from build123d import *

# Parameters (mm, degrees)
SKETCH_3_R          = 23.4
EXTRUDE_1_DEPTH     = 7.81
SKETCH_2_R          = 21.6
CUT_EXTRUDE_1_DEPTH = 2.1
CUT_EXTRUDE_START   = 2.1
CUT_EXTRUDE_2_DEPTH = 3.2
CUT_EXTRUDE_START_2 = 7.81
SKETCH_4_R          = 1.49999954
SKETCH_4_R_2        = 1.25000004
CUT_EXTRUDE_5_DEPTH = 8.81
SKETCH_5_R          = 1.65
CUT_EXTRUDE_6_DEPTH = 0.9
SKETCH_6_R          = 2.35
CUT_EXTRUDE_7_DEPTH = 2.7
CUT_EXTRUDE_START_3 = 5.3
SKETCH_7_R          = 3.2
CUT_EXTRUDE_8_DEPTH = 1
CHAMFER_1_SIZE      = 1
CHAMFER_2_SIZE      = 0.25
CHAMFER_3_SIZE      = 0.2


with BuildPart() as part:
    # 草图3 → 凸台-拉伸1 (new body)
    with BuildSketch(Plane.XY):
        with Locations((100.000148425, 100.000129687)):
            Circle(SKETCH_3_R)
    extrude(amount=EXTRUDE_1_DEPTH)

    # 草图2 → 切除-拉伸1 (cut)
    with BuildSketch(Plane.XY):
        with Locations((100.000148425, 100.000129687)):
            Circle(SKETCH_2_R)
    extrude(amount=CUT_EXTRUDE_1_DEPTH, mode=Mode.SUBTRACT)

    # 草图1 → 切除-拉伸2 (cut)
    with BuildSketch(Plane.XY.offset(CUT_EXTRUDE_START)):
        with BuildLine():
            Line((112.259115553, 115.826027875), (111.656637713, 115.826027875))
            Line((111.656637713, 115.826027875), (97.599477613, 115.826027875))
            Line((97.599477613, 115.826027875), (96.687659742, 115.826027875))
            ThreePointArc((96.687659742, 115.826027875), (96.087351408, 115.611111205), (95.759847053, 115.064027875))
            Line((95.759847053, 115.064027875), (95.759847053, 109.857027875))
            Line((95.759847053, 109.857027875), (95.759847053, 105.158027875))
            ThreePointArc((95.759847053, 105.158027875), (95.387872666, 104.260002263), (94.489847053, 103.888027875))
            Line((94.489847053, 103.888027875), (83.186847053, 103.888027875))
            ThreePointArc((83.186847053, 103.888027875), (82.288821441, 103.516053487), (81.916847053, 102.618027875))
            Line((81.916847053, 102.618027875), (81.916847053, 92.712027875))
            ThreePointArc((81.916847053, 92.712027875), (82.288821441, 91.814002263), (83.186847053, 91.442027875))
            Line((83.186847053, 91.442027875), (92.965847053, 91.442027875))
            ThreePointArc((92.965847053, 91.442027875), (94.021841281, 91.231977601), (94.917069973, 90.633804955))
            Line((94.917069973, 90.633804955), (95.676425833, 89.874449095))
            ThreePointArc((95.676425833, 89.874449095), (96.208135359, 89.078689918), (96.394847053, 88.140027875))
            Line((96.394847053, 88.140027875), (96.394847053, 81.461633815))
            ThreePointArc((96.394847053, 81.461633815), (96.427853197, 81.29569991), (96.521847053, 81.155027875))
            ThreePointArc((96.521847053, 81.155027875), (96.943861908, 80.87304655), (97.441662377, 80.774027875))
            Line((97.441662377, 80.774027875), (97.537847053, 80.774027875))
            Line((97.537847053, 80.774027875), (101.772425833, 80.774027875))
            Line((101.772425833, 80.774027875), (102.236847053, 80.774027875))
            ThreePointArc((102.236847053, 80.774027875), (102.865464982, 81.034409947), (103.125847053, 81.663027875))
            Line((103.125847053, 81.663027875), (103.125847053, 83.695027875))
            ThreePointArc((103.125847053, 83.695027875), (103.349031686, 84.233843243), (103.887847053, 84.457027875))
            Line((103.887847053, 84.457027875), (111.60403053, 84.457027875))
            ThreePointArc((111.60403053, 84.457027875), (112.336497489, 84.602724612), (112.957452993, 85.017633815))
            Line((112.957452993, 85.017633815), (117.811624454, 89.871805276))
            ThreePointArc((117.811624454, 89.871805276), (118.408450098, 90.766392606), (118.618000745, 91.821179725))
            Line((118.618000745, 91.821179725), (118.618000745, 108.839))
            Line((118.618000745, 108.839), (118.618000745, 109.460547459))
            ThreePointArc((118.618000745, 109.460547459), (118.537945969, 109.810671539), (118.33936792, 110.109941312))
            Line((118.33936792, 110.109941312), (117.729, 110.744000093))
            Line((117.729, 110.744000093), (115.585546543, 112.887726165))
            ThreePointArc((115.585546543, 112.887726165), (114.325244429, 114.275507158), (112.941853583, 115.540626625))
            ThreePointArc((112.941853583, 115.540626625), (112.628834267, 115.751145515), (112.259115553, 115.826027875))
        make_face()
    extrude(amount=CUT_EXTRUDE_2_DEPTH, mode=Mode.SUBTRACT)

    # 草图4 → 切除-拉伸5 (cut, through all)
    with BuildSketch(Plane.XY.offset(CUT_EXTRUDE_START_2)):
        with Locations((85.217, 99.949)):
            Circle(SKETCH_4_R)
        with Locations((93.13750232, 88.11380142)):
            Circle(SKETCH_4_R_2)
        with Locations((93.13749978, 111.8861999)):
            Circle(SKETCH_4_R_2)
    extrude(amount=-CUT_EXTRUDE_5_DEPTH, mode=Mode.SUBTRACT)

    # 草图5 → 切除-拉伸6 (cut)
    with BuildSketch(Plane.XY.offset(CUT_EXTRUDE_START_2)):
        with Locations((85.217, 99.949)):
            Circle(SKETCH_5_R)
    extrude(amount=-CUT_EXTRUDE_6_DEPTH, mode=Mode.SUBTRACT)

    # 草图6 → 切除-拉伸7 (cut)
    with BuildSketch(Plane.XY.offset(CUT_EXTRUDE_START_2)):
        with Locations((93.13749978, 111.8861999)):
            Circle(SKETCH_6_R)
        with Locations((93.13750232, 88.11380142)):
            Circle(SKETCH_6_R)
    extrude(amount=-CUT_EXTRUDE_7_DEPTH, mode=Mode.SUBTRACT)

    # 草图7 → 切除-拉伸8 (cut)
    with BuildSketch(Plane.XY.offset(CUT_EXTRUDE_START_3)):
        with Locations((100.018718989, 99.944811263)):
            Circle(SKETCH_7_R)
    extrude(amount=CUT_EXTRUDE_8_DEPTH, mode=Mode.SUBTRACT)

    # 倒角1
    chamfer_1_edges = [part.edges().sort_by_distance(p)[0] for p in [
        (76.600148425, 100.000129687, 7.81),
    ]]
    chamfer(chamfer_1_edges, length=CHAMFER_1_SIZE)

    # 倒角2
    chamfer_2_edges = [part.edges().sort_by_distance(p)[0] for p in [
        (76.600148425, 100.000129687, 0),
        (78.400148425, 100.000129687, 0),
    ]]
    chamfer(chamfer_2_edges, length=CHAMFER_2_SIZE)

    # 倒角3
    chamfer_3_edges = [part.edges().sort_by_distance(p)[0] for p in [
        (90.78749978, 111.8861999, 7.81),
        (90.78750232, 88.11380142, 7.81),
        (96.818718989, 99.944811263, 5.3),
    ]]
    chamfer(chamfer_3_edges, length=CHAMFER_3_SIZE)


solid = part.part
Geometry: final body of the model. Coordinates: model frame, mm. A direction names the side the tool comes from. Round coordinates to 2 decimals unless told otherwise and drop trailing zeros. Loops run counter-clockwise (first coordinate to the right, second up) from the corner with the lowest first, then second, coordinate; pieces in that order, holes last. Notation, with made-up numbers: (0.5, 5.25) -> (59.5, 5.25) arc R15 cw to (59.5, 21.25) -> close; hole circle Ø11 at (64.5, -12.5). An arc over 180 degrees is marked (long way). One line per question, with ' | ' between items. Start each with the question number.
1. Line query: line 1 along X through (y, z) = (109, 4.25); line 2 along Y through (x, z) = (110, 1); line 3 along Z through (x, y) = (79, 102). Output: solid intervals per line, ascending. Write a range as [from, to].
2. Set-up query: faces 1 (the face through (86.023, 101.214, 6.116)), 2 (the face through (95.31, 110.99, 6.38)), 3 (the face through (94.008, 91.238, 3.678)). Return all of +Z, -Z, +X, -X, +Y, -Y with unobstructed straight access to the full face (end or side cutting, diameter ignored); none if empty.
3. Section A-A on z = 3.5. Count the separate pieces of the cut face and the enclosed holes in it, and give its area (3 significant figures).
4. Contact query for flat-ended pins moving along their axis: pin 1 (2.5 mm diameter, centred on y = 97.5, z = 3.5, fed in from +X); pin 2 (4 mm diameter, centred on x = 85.217, y = 99.949, fed in from -Z); pin 3 (3.5 mm diameter, centred on x = 101, z = 4.5, fed in from -Y). Output: stop coordinate, or through.
5. Section B-B on z = 1. Output: boundary loops of the cut face in (x, y).
Returned:
1) line 1: x = [78.4, 95.76], [118.62, 121.6] | line 2: y = [78.84, 80.85], [119.15, 121.16] | line 3: z = [2.1, 7.81]
2) face 1: +Z, -Z | face 2: +Z | face 3: -Z
3) separate pieces: 1 | enclosed holes: 3 | area: 836 mm2
4) pin 1: stops at x = 123.37 | pin 2: stops at z = 5.3 | pin 3: stops at y = 76.6
5) outline: circle Ø46.8 at (100, 100); hole circle Ø43.2 at (100, 100)
